from build123d import *

# Parameters (mm, degrees)
BOSS_EXTRUDE1_DEPTH  = 133.35
SKETCH2_W            = 6.06425
SKETCH2_H            = 5.11175
BOSS_EXTRUDE2_DEPTH  = 1.5875
FILLET1_R            = 3.175
FILLET1_OF_MIRROR1_R = 3.175
FILLET2_R            = 0.635


with BuildPart() as part:
    # Sketch1 → Boss-Extrude1 (new body)
    with BuildSketch(Plane.XY):
        Polygon((0.142875, 3.667125), (3.032125, 3.667125), (3.032125, 1.905), (3.032125, 0.142875), (0.142875, 0.142875), (0.142875, 1.905), align=None)
    extrude(amount=BOSS_EXTRUDE1_DEPTH)

    # Sketch2 → Boss-Extrude2 (add)
    with BuildSketch(Plane.XY.offset(133.35)):
        with Locations((1.5875, 2.69875)):
            Rectangle(SKETCH2_W, SKETCH2_H)
    boss_extrude2 = extrude(amount=BOSS_EXTRUDE2_DEPTH)

    # Fillet1
    # the kernel refuses this fillet: 3.175 mm, written as the material it takes off along each edge
    with BuildSketch(Plane(origin=(-1.444625, 5.254625, 125.4125), x_dir=(0, -1, 0), z_dir=(0, 0, 1))) as fillet1_piece_1:
        with BuildLine():
            CenterArc((FILLET1_R, FILLET1_R), FILLET1_R, 180, 90)
            Line((0, FILLET1_R), (0, 0))
            Line((0, 0), (FILLET1_R, 0))
        make_face()
    extrude(amount=17.4625, mode=Mode.SUBTRACT)
    with BuildSketch(Plane(origin=(4.619625, 5.254625, 125.4125), x_dir=(0, -1, 0), z_dir=(0, 0, 1))) as fillet1_piece_2:
        with BuildLine():
            CenterArc((FILLET1_R, -FILLET1_R), FILLET1_R, 90, 90)
            Line((0, -FILLET1_R), (0, 0))
            Line((0, 0), (FILLET1_R, 0))
        make_face()
    extrude(amount=17.4625, mode=Mode.SUBTRACT)

    # Mirror1: Boss-Extrude2 across plane
    add(boss_extrude2.mirror(Plane.XY.offset(66.675)))

    # Fillet1 of Mirror1
    # the kernel refuses this fillet: 3.175 mm, written as the material it takes off along each edge
    with BuildSketch(Plane(origin=(-1.444625, 5.254625, 7.9375), x_dir=(0, -1, 0), z_dir=(0, 0, -1))) as fillet1_of_mirror1_piece_1:
        with BuildLine():
            CenterArc((FILLET1_OF_MIRROR1_R, -FILLET1_OF_MIRROR1_R), FILLET1_OF_MIRROR1_R, 90, 90)
            Line((0, -FILLET1_OF_MIRROR1_R), (0, 0))
            Line((0, 0), (FILLET1_OF_MIRROR1_R, 0))
        make_face()
    extrude(amount=17.4625, mode=Mode.SUBTRACT)
    with BuildSketch(Plane(origin=(4.619625, 5.254625, 7.9375), x_dir=(0, -1, 0), z_dir=(0, 0, -1))) as fillet1_of_mirror1_piece_2:
        with BuildLine():
            CenterArc((FILLET1_OF_MIRROR1_R, FILLET1_OF_MIRROR1_R), FILLET1_OF_MIRROR1_R, 180, 90)
            Line((0, FILLET1_OF_MIRROR1_R), (0, 0))
            Line((0, 0), (FILLET1_OF_MIRROR1_R, 0))
        make_face()
    extrude(amount=17.4625, mode=Mode.SUBTRACT)

    # Fillet2
    fillet2_edges = [part.edges().sort_by_distance(p)[0] for p in [
        (3.032125, 3.667125, 66.675),
        (0.142875, 3.667125, 66.675),
    ]]
    fillet(fillet2_edges, radius=FILLET2_R)


solid = part.part
For this review, take the finished solid that the model builds, in its own axes (mm). A direction names the side the tool comes from. Round coordinates to 2 decimals unless told otherwise and drop trailing zeros. Write each loop counter-clockwise with the first axis right and the second up, starting at its lowest first coordinate (ties: lowest second). Pieces come first, ordered by that corner, then holes. Notation, with made-up numbers: (-24, 40) - (1, 40) arc R4 ccw to (1, 47) - close; hole circle Ø2 at (73, 59). An arc over 180 degrees is marked (long way). Use a Markdown table: item, result.
Q1. We need section A-A (z = 56.5). Give the boundary of the cut face in (x, y) (3 decimals), plus the area to 3 significant figures.
Derived:
| item | result |
|---|---|
| outline | (0.143, 0.143) - (3.032, 0.143) - (3.032, 3.032) arc R0.635 ccw to (2.397, 3.667) - (0.778, 3.667) arc R0.635 ccw to (0.143, 3.032) - close |
| area | 10.0 mm2 |
Q2. Wall thickness on line 1 along Z through (x, y) = (1.75, 4.8); line 2 along X through (y, z) = (0.45, 12); line 3 along Y through (x, z) = (0.75, 58): over which ranges is each line inside the solid? List them lowest first.
Derived:
| item | result |
|---|---|
| line 1 | z = -1.59 to 0, 133.35 to 134.94 |
| line 2 | x = 0.14 to 3.03 |
| line 3 | y = 0.14 to 3.67 |
Q3. Clearance check with flat-ended pins moving along their axes: pin 1 (2.5 mm diameter, centred on y = 2, z = 33.5, fed in from +X); pin 2 (3 mm diameter, centred on y = 1.5, z = 72.5, fed in from -X); pin 3 (1.5 mm diameter, centred on x = 3, z = 34, fed in from +Y). State where each tip first meets the part, or that it passes through.
Derived:
| item | result |
|---|---|
| pin 1 | stops at x = 3.03 |
| pin 2 | stops at x = 0.14 |
| pin 3 | stops at y = 3.67 |
Q4. We need section B-B (y = 4.45). Give the boundary of the cut face in (x, z).
Derived:
| item | result |
|---|---|
| outline | (-0.38, -1.59) - (3.56, -1.59) - (3.56, 0) - (-0.38, 0) - close; (-0.38, 133.35) - (3.56, 133.35) - (3.56, 134.94) - (-0.38, 134.94) - close |
Q5. The part is to be moulded in two halves that separate along Z. For faces 1 (the flat face through (2, 4, 133.35)), 2 (the flat face through (2, 2, 134.938)), 3 (the flat face through (2, 0.143, 68)), say which applies: pulls with the +Z half, pulls with the -Z half, needs draft (parallel to the pull), parting line crosses it, or undercut.
Derived:
| item | result |
|---|---|
| face 1 | undercut |
| face 2 | pulls with the +Z half |
| face 3 | needs draft |
Q6. Machinability: for faces 4 (the flat face through (3.032, 2, 66)), 5 (the flat face through (2, 4, 0)), 6 (the flat face through (0.143, 2, 66)), which of the approach directions +Z, -Z, +X, -X, +Y, -Y give a long, thin tool a straight path to every point of the face, cutting with its end or side? Answer none if there is none.
Derived:
| item | result |
|---|---|
| face 4 | +X, +Y, -Y |
| face 5 | +Y |
| face 6 | -X, +Y, -Y |
